from build123d import *

# Parameters (mm, degrees)
F0_R     = 27.5
F0_R_2   = 24.5
F1_DEPTH = 3
F0_R_3   = 22.5
F2_DEPTH = 18
F3_R     = 1
F4_R     = 1.5
F5_R     = 0.99999
F7_D     = 6
F7_DEPTH = 25
F7_TIP   = 1.8025818571


# Not quite as in the source:
# - a fillet or chamfer is up to 0.001 mm smaller than in the source, because OpenCascade refuses the exact size


with BuildPart() as f1:
    # F0 (on Top) → F1 (new body)
    with BuildSketch(Plane.XY):
        Circle(F0_R)
        Circle(F0_R_2, mode=Mode.SUBTRACT)
    extrude(amount=F1_DEPTH)

    # F0 (on Top) → F2 (join)
    with BuildSketch(Plane.XY):
        Circle(F0_R_2)
        Circle(F0_R_3, mode=Mode.SUBTRACT)
    extrude(amount=F2_DEPTH)

    # F3
    f3_edges = [f1.edges().sort_by_distance(p)[0] for p in [
        (-27.5, 0, 0),
        (-22.5, 0, 0),
    ]]
    fillet(f3_edges, radius=F3_R)

    # F4
    f4_edges = [f1.edges().sort_by_distance(p)[0] for p in [
        (-27.5, 0, 3),
    ]]
    fillet(f4_edges, radius=F4_R)

    # F5 (radius 1 in the source; OpenCascade refuses exactly that, so slightly less here)
    f5_edges = [f1.edges().sort_by_distance(p)[0] for p in [
        (-22.5, 0, 18),
        (-24.5, 0, 18),
    ]]
    fillet(f5_edges, radius=F5_R)

    # F7 (one way)
    with BuildSketch(Plane.YZ):
        with Locations((0, 9.8607558757)):
            Circle(F7_D / 2)
    extrude(amount=-F7_DEPTH, mode=Mode.SUBTRACT)
    with Locations(Plane.YZ):
        with Locations((0, 9.8607558757)):
            with Locations((0, 0, -(F7_DEPTH + F7_TIP / 2))):  # 118° drill point
                Cone(0, F7_D / 2, F7_TIP, mode=Mode.SUBTRACT)


solid = f1.part
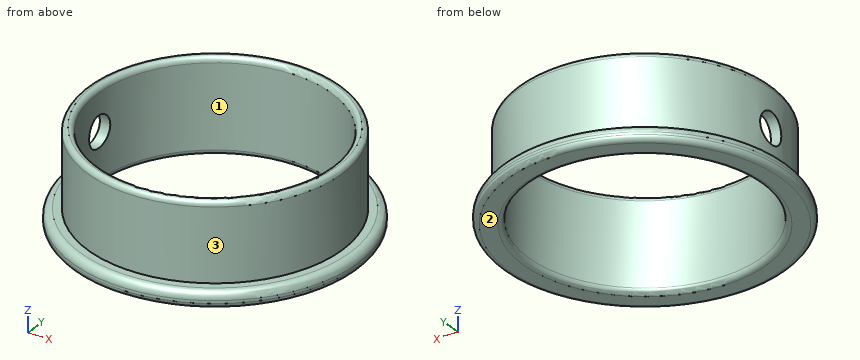
Design review of the part built by this model. Coordinates are the model's own, in mm. Face numbers are marked on the shaded views. Coordinates: 2 decimals unless noted, no trailing zeros. Loops run counter-clockwise (first coordinate to the right, second up) from the corner with the lowest first, then second, coordinate; pieces in that order, holes last. Notation, with made-up numbers: (39, 27.5) -> (53, 27.5) arc R32 ccw to (53, 57.5) -> close; hole circle Ø3 at (70.5, 22). An arc over 180 degrees is marked (long way). Use a Markdown table: item, result. Add a question column.
Item 1: Wall thickness on L1, parallel to Y at x = 0, z = 5; L2, parallel to Y at x = 10, z = 8.75: over which ranges is each line inside the solid? List them lowest first. Write a range as from..to.
Item 2: We need section C-C, the plane z = 15.5. Write out the cut boundary in (x, y), and give its area (3 significant figures).
Item 3: Clearance check with flat-ended pins moving along their axes: P1, Ø6, axis at y = 10.5, z = 13, coming from the -X side; P2, Ø5.5, axis at y = 0, z = 9.86, coming from the -X side; P3, Ø4, axis at y = -13.5, z = 13, coming from the -X side; P4, Ø8, axis at x = -17, y = -15, coming from the -Z side. State where each tip first meets the part, or that it passes through.
Item 4: The part is to be moulded in two halves that separate along X. For the marked faces 1, 2 and 3, say which applies: +X half, -X half, draft (parallel to the pull), parting line (faces both ways), or undercut.
Item 5: We need section D-D, the plane z = 10.5. Write out the cut boundary in (x, y), and give its area (3 significant figures).
Item 6: We need section B-B, the plane y = 0. Count the separate pieces of the cut face and the enclosed holes in it, and give its area (3 significant figures).
Numbers:
| question | item | result |
|---|---|---|
| 1 | L1 | y = -24.5..-22.5, 22.5..24.5 |
| 1 | L2 | y = -22.37..-20.16, 20.16..22.37 |
| 2 | outline | circle Ø49 at (0, 0); hole circle Ø45 at (0, 0) |
| 2 | area | 295 mm^2 |
| 3 | P1 | stops at x = -23.32 |
| 3 | P2 | stops at x = 22.33 |
| 3 | P3 | stops at x = -21.63 |
| 3 | P4 | stops at z = 0 |
| 4 | face 1 | undercut |
| 4 | face 2 | draft |
| 4 | face 3 | parting line |
| 5 | outline | (-24.32, -2.93) arc R24.5 ccw (long way) to (-24.32, 2.93) -> (-22.31, 2.93) arc R22.5 cw (long way) to (-22.31, -2.93) -> close |
| 5 | area | 284 mm^2 |
| 6 | separate pieces | 3 |
| 6 | enclosed holes | 0 |
| 6 | area | 75.3 mm^2 |
